Design review of the part shown in the three views and the two pictorial views. Dimensions are in mm from the part's minimum x, y and z. A direction names the side the tool comes from. Give positions to 0.01 mm unless a question says otherwise; leave off trailing zeros. Loops run counter-clockwise (first coordinate to the right, second up) from the corner with the lowest first, then second, coordinate; pieces in that order, holes last.
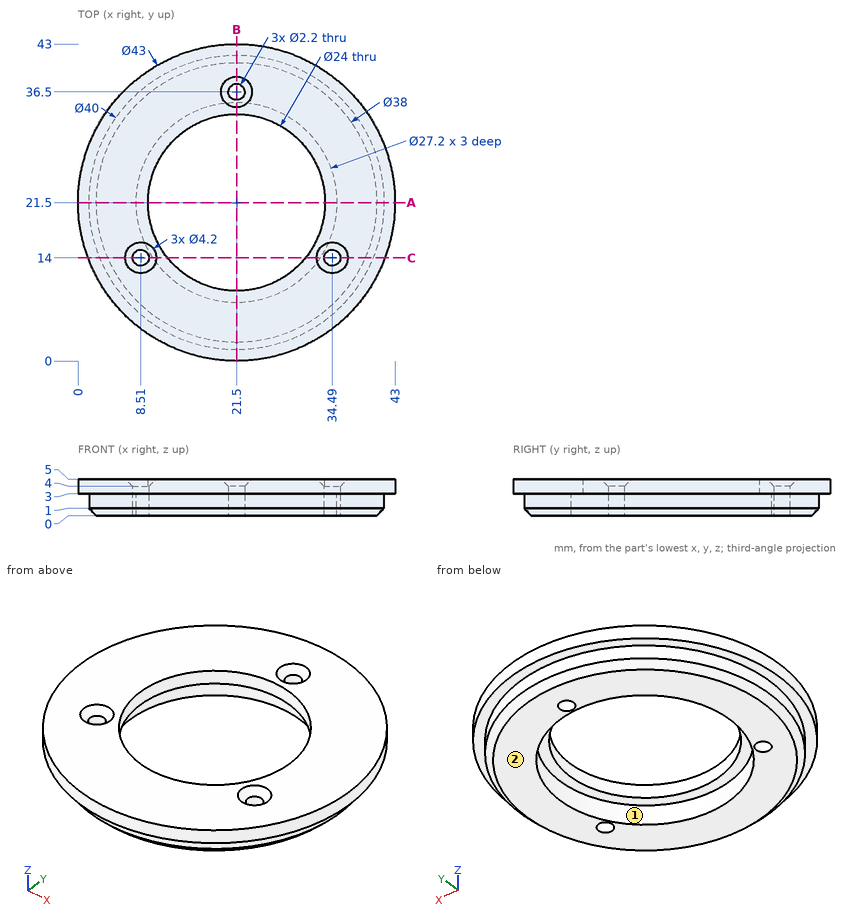
Q1. Take a section at A-A (y = 21.5). Give the boundary of the cut face in (x, z), plus the area to 3 significant figures.
Results:
outline: (0, 3) - (1.5, 3) - (1.5, 1) - (2.5, 0) - (7.9, 0) - (7.9, 3) - (9.5, 3) - (9.5, 5) - (0, 5) - close; (33.5, 3) - (35.1, 3) - (35.1, 0) - (40.5, 0) - (41.5, 1) - (41.5, 3) - (43, 3) - (43, 5) - (33.5, 5) - close
area: 75.4 mm2
Q2. Tool access review of the marked faces 1 and 2: name each direction out of +Z, -Z, +X, -X, +Y, -Y from which nothing blocks a thin tool from reaching the whole face with its end or side.
Results:
face 1: -Z
face 2: -Z, +X, -X, +Y, -Y
Q3. Wall thickness on line 1 (X direction, y = 21.5, z = 2); line 2 (X direction, y = 21, z = 3.65) (1 decimal); line 3 (Z direction, x = 9, y = 16.5): over which ranges is each line inside the solid? List them lowest first.
Results:
line 1: x = 1.5 to 7.9, 35.1 to 41.5
line 2: x = 0 to 9.5, 33.5 to 43
line 3: z = 3 to 5
Q4. Insertion check: pin 1 (3.5 mm diameter, centred on x = 34.49, y = 14, fed in from +Z); pin 2 (5 mm diameter, centred on x = 35.5, y = 11, fed in from -Z); pin 3 (3 mm diameter, centred on y = 22.5, z = 2.5, fed in from +X); pin 4 (3 mm diameter, centred on y = 29.5, z = 1, fed in from +X) (1 decimal). Each pin has a flat end and moves straight along its axis. Give the tip position at first contact, or say it passes through.
Results:
pin 1: stops at z = 4.65
pin 2: stops at z = 0
pin 3: stops at x = 43
pin 4: stops at x = 40.4
Q5. Take a section at C-C (y = 14). Give the number of separate pieces and of enclosed holes in the cut face.
Results:
separate pieces: 4
enclosed holes: 0
Q6. Take a section at B-B (x = 21.5). Give the boundary of the cut face in (y, z).
Results:
outline: (0, 3) - (1.5, 3) - (1.5, 1) - (2.5, 0) - (7.9, 0) - (7.9, 3) - (9.5, 3) - (9.5, 5) - (0, 5) - close; (33.5, 3) - (35.1, 3) - (35.1, 0) - (35.4, 0) - (35.4, 4) - (34.4, 5) - (33.5, 5) - close; (37.6, 0) - (40.5, 0) - (41.5, 1) - (41.5, 3) - (43, 3) - (43, 5) - (38.6, 5) - (37.6, 4) - close
